Here's how the part is built. I have some questions about the finished solid (model axes, mm). A direction names the side the tool comes from. Coordinates: 2 decimals unless noted, no trailing zeros. Loops run counter-clockwise (first coordinate to the right, second up) from the corner with the lowest first, then second, coordinate; pieces in that order, holes last.
from build123d import *

# Parameters (mm, degrees)
IZIM1_W                     = 38
IZIM1_H                     = 54
Y_KSEKLIK_EKSTR_ZYON1_DEPTH = 8
IZIM2_W                     = 8
IZIM2_H                     = 4
KES_EKSTR_ZYON1_DEPTH       = 67.513156593
RADYUS1_R                   = 3
RADYUS2_R                   = 10
IZIM4_R                     = 2.5
KES_EKSTR_ZYON2_DEPTH       = 67.513156593
Y_KSEKLIK_EKSTR_ZYON2_DEPTH = 8
RADYUS3_R                   = 10
IZIM6_R                     = 14
Y_KSEKLIK_EKSTR_ZYON3_DEPTH = 8
IZIM7_R                     = 5
KES_EKSTR_ZYON3_DEPTH       = 88.229582138
FEDER2_REACH                = 76.007
IZIM8_WALL_W                = 184.841662432
IZIM8_WALL_H                = 6


with BuildPart() as part:
    # Çizim1 → Yükseklik-Ekstrüzyon1 (new body)
    with BuildSketch(Plane(origin=(0, 0, 0), x_dir=(1, 0, 0), z_dir=(0, 1, 0))):
        with Locations((-19, 27)):
            Rectangle(IZIM1_W, IZIM1_H)
    extrude(amount=Y_KSEKLIK_EKSTR_ZYON1_DEPTH)

    # Çizim2 → Kes-Ekstrüzyon1 (cut, through all)
    with BuildSketch(Plane.XY):
        with Locations((-4, 6)):
            Rectangle(IZIM2_W, IZIM2_H)
    extrude(amount=-KES_EKSTR_ZYON1_DEPTH, mode=Mode.SUBTRACT)

    # Radyus1
    radyus1_edges = [part.edges().sort_by_distance(p)[0] for p in [
        (-8, 4, -27),
    ]]
    fillet(radyus1_edges, radius=RADYUS1_R)

    # Radyus2
    radyus2_edges = [part.edges().sort_by_distance(p)[0] for p in [
        (-38, 4, 0),
        (-38, 4, -54),
    ]]
    fillet(radyus2_edges, radius=RADYUS2_R)

    # Çizim4 → Kes-Ekstrüzyon2 (cut, through all)
    with BuildSketch(Plane(origin=(0, 8, 0), x_dir=(1, 0, 0), z_dir=(0, 1, 0))):
        with Locations(Location((-28, 44, 0), (0, 0, 270))):
            Circle(IZIM4_R)
        with Locations(Location((-28, 10, 0), (0, 0, 270))):
            Circle(IZIM4_R)
    extrude(amount=-KES_EKSTR_ZYON2_DEPTH, mode=Mode.SUBTRACT)

    # Çizim5 → Yükseklik-Ekstrüzyon2 (add)
    with BuildSketch(Plane(origin=(-8, 0, 0), x_dir=(0, 0, -1), z_dir=(1, 0, 0))):
        with BuildLine():
            Line((14, 43), (14, 8))
            Line((14, 8), (42, 8))
            Line((42, 8), (42, 43))
            ThreePointArc((42, 43), (28, 57), (14, 43))
        make_face()
    extrude(amount=-Y_KSEKLIK_EKSTR_ZYON2_DEPTH)

    # Radyus3
    radyus3_edges = [part.edges().sort_by_distance(p)[0] for p in [
        (-12, 8, -42),
        (-12, 8, -14),
    ]]
    fillet(radyus3_edges, radius=RADYUS3_R)

    # Çizim6 → Yükseklik-Ekstrüzyon3 (add)
    with BuildSketch(Plane(origin=(-8, 0, 0), x_dir=(0, 0, -1), z_dir=(1, 0, 0))):
        with Locations((28, 43)):
            Circle(IZIM6_R)
    extrude(amount=Y_KSEKLIK_EKSTR_ZYON3_DEPTH)

    # Çizim7 → Kes-Ekstrüzyon3 (cut, through all)
    with BuildSketch(Plane(origin=(0, 0, 0), x_dir=(0, 0, -1), z_dir=(1, 0, 0))):
        with Locations((28, 43)):
            Circle(IZIM7_R)
    extrude(amount=-KES_EKSTR_ZYON3_DEPTH, mode=Mode.SUBTRACT)

    # Çizim8 wall → Feder2 (add, up to next)
    with BuildSketch(Plane(origin=(-27, 21.5, -28), x_dir=(0.631672951162, 0.775234985517, 0), z_dir=(-0.775234985517, 0.631672951162, 0)), mode=Mode.PRIVATE) as feder2_sk1:
        Rectangle(IZIM8_WALL_W, IZIM8_WALL_H)
    feder2_tool1 = extrude(feder2_sk1.sketch, amount=-FEDER2_REACH, mode=Mode.PRIVATE) - part.part
    add(feder2_tool1.solids().sort_by_distance((-27, 21.5, -28))[0])


solid = part.part
Q1. For faces 1 (the flat face through (-12, 30, -42)), 2 (the flat face through (-3, 4, -27)), 3 (the flat face through (-22, 17, -31)), 4 (the flat face through (-22, 17, -25)), which set-ups out of +Z, -Z, +X, -X, +Y, -Y let a thin tool reach every point of the face, with its end or its side?
Q2. We'd pull the mould along Y, two halves only. Please class faces 5 (the flat face through (-19, 0, -27)), 6 (the cylindrical face through (-25.52, 4.06, -10.33)), 7 (the cylindrical face through (-6.33, 56.88, -26.18)): pulls with the +Y half, pulls with the -Y half, needs draft (parallel to the pull), parting line crosses it, or undercut.
Q3. Suppose I cut it at D-D on x = -18.5. Write out the boundary of the cut face in (y, z).
Q4. Will these pins go through, and if not, where does the flat tip stop? P1, Ø4.5, axis at x = -28, z = -44, coming from the -Y side; P2, Ø2.5, axis at x = -12.5, y = 26.5, coming from the +Z side; P3, Ø1, axis at x = -5.5, y = 39.5, coming from the -Z side; P4, Ø4, axis at x = -13, y = 25.5, coming from the -Z side.
Q5. Suppose I cut it at C-C on y = 41. Write out the boundary of the cut face in (x, z).
Q6. Please list where these lines run through material, in increasing order: probe 1 along Y at (x, z) = (-2, -31); probe 2 along X at (y, z) = (7, -14.5); probe 3 along Y at (x, z) = (-29, -40.5).
Q7. Suppose I cut it at B-B on x = -4. Write out the boundary of the cut face in (y, z).
Q8. Suppose I cut it at A-A on z = -28. Write out the boundary of the cut face in (x, y), and give its area (3 significant figures).
Check values:
1. face 1: -Z, +X, -X, +Y
1. face 2: +Z, -Z, +X
1. face 3: -Z, -X, +Y
1. face 4: +Z, -X, +Y
2. face 5: pulls with the -Y half
2. face 6: needs draft
2. face 7: undercut
3. outline: (0, -54) - (8, -54) - (8, -31) - (31.93, -31) - (31.93, -25) - (8, -25) - (8, 0) - (0, 0) - close
4. P1: passes through
4. P2: stops at z = -14
4. P3: stops at z = -41.67
4. P4: stops at z = -42
5. outline: (-16, -42) - (-8, -42) - (-8, -41.86) - (0, -41.86) - (0, -32.58) - (-16, -32.58) - close; (-16, -23.42) - (0, -23.42) - (0, -14.14) - (-8, -14.14) - (-8, -14) - (-16, -14) - close
6. probe 1: y = 0 to 4, 29.33 to 39, 47 to 56.67
6. probe 2: x = -38 to -8
6. probe 3: y = 0 to 8
7. outline: (0, -54) - (4, -54) - (4, 0) - (0, 0) - close; circle Ø28 at (43, -28); hole circle Ø10 at (43, -28)
8. outline: (-38, 0) - (0, 0) - (0, 4) - (-5, 4) arc R3 cw to (-8, 7) - (-8, 29) - (0, 29) - (0, 38) - (-16, 38) - (-16, 35) - (-38, 8) - close; (-16, 48) - (0, 48) - (0, 57) - (-16, 57) - close
8. area: 1,030 mm2
